Answer from the drawing. Dimensions are ordinates in mm from the lowest x, y and z of the part. A direction names the side the tool comes from. Coordinates: 2 decimals unless noted, no trailing zeros. Write each loop counter-clockwise with the first axis right and the second up, starting at its lowest first coordinate (ties: lowest second). Pieces come first, ordered by that corner, then holes. Notation, with made-up numbers: (22.5, -9.75) -> (54.5, -9.75) arc R24 cw to (54.5, 6.25) -> close; hole circle Ø4 at (55, 47). An arc over 180 degrees is marked (long way). Answer as a JSON object with one key per item and string values. Group by question number.
(1) Which of the six approach directions +Z, -Z, +X, -X, +Y, -Y give full straight-line access (tool end or side, diameter ignored) to the marked faces 1, 2 and 3?
(2) Straight lines are drawn through the part: L1, parallel to Z at x = 10, y = 19; L2, parallel to X at y = 22, z = 10; L3, parallel to Y at x = 10, z = 6. For each, find the intervals that lie inside material, in ascending order.
(3) For a pull along X with two mould halves and no side action, classify the marked faces 4, 5 and 6 as +X half, -X half, draft (parallel to the pull), parting line (faces both ways), or undercut.
(4) Find section D-D (y = 7.25). Give the vertices of the cut face in (x, z).
(5) Find section B-B (z = 5.5). Give the vertices of the cut face in (x, y), then the cut area to 3 significant figures.
(6) Find section C-C (x = 18). Give the vertices of the cut face in (y, z), then the cut area to 3 significant figures.
(7) Find section A-A (y = 21.5). Give the vertices of the cut face in (x, z) (1 decimal).
(8) Flat-ended cylindrical pins translate along their axes: P1, Ø3, axis at x = 10, y = 22, coming from the -Z side; P2, Ø2, axis at x = 11, z = 9, coming from the +Y side; P3, Ø1.2, axis at x = 10, y = 21.5, coming from the -Z side; P4, Ø6, axis at y = 22, z = 4, coming from the -X side (1 decimal). Find the tip coordinate at first contact, or state that the pin passes through.
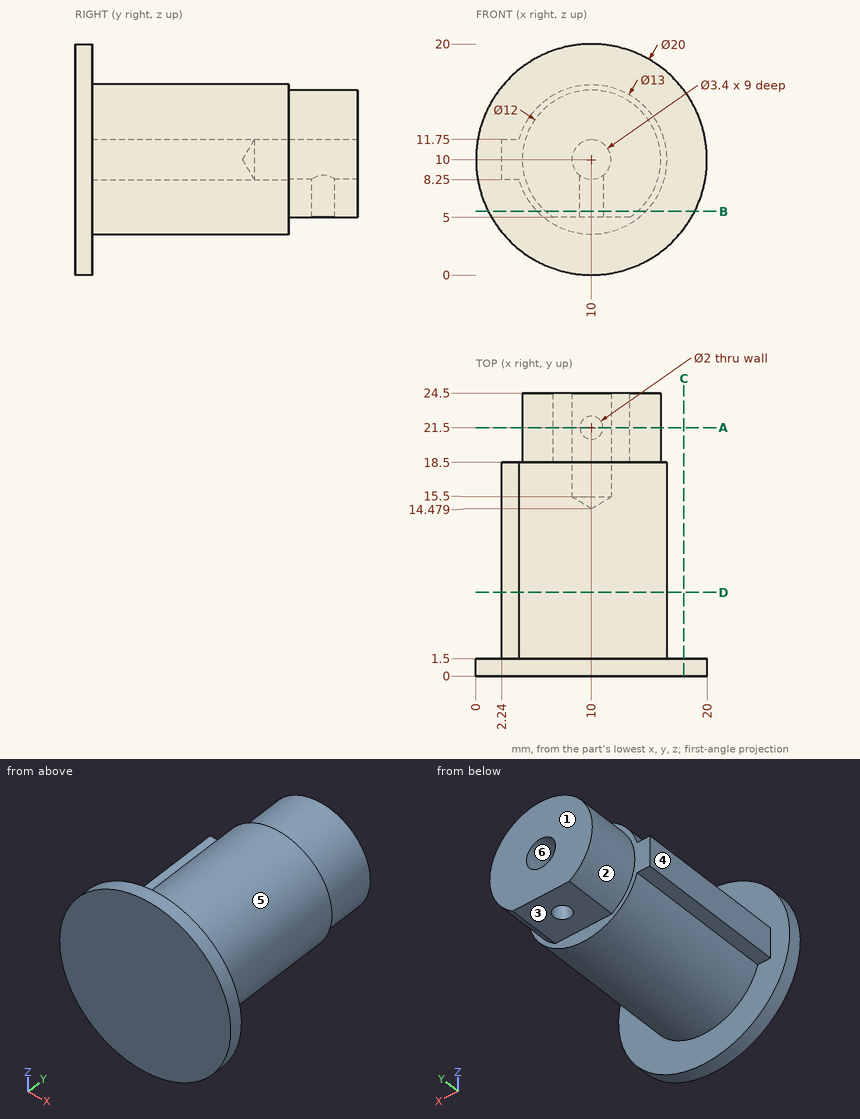
Results below:
{
 "1": {"face 1": "+Z, -Z, +X, -X, +Y", "face 2": "+Y", "face 3": "-Z, +X, -X, +Y"},
 "2": {"L1": "z = 5 to 8.3, 11.7 to 16", "L2": "x = 4 to 8.3, 11.7 to 16", "L3": "y = 0 to 20.5, 22.5 to 24.5"},
 "3": {"face 4": "-X half", "face 5": "parting line", "face 6": "undercut"},
 "4": {"outline": "(2.24, 8.25) -> (3.74, 8.25) arc R6.5 ccw (long way) to (3.74, 11.75) -> (2.24, 11.75) -> close"},
 "5": {"outline": "(1.07, 0) -> (18.93, 0) -> (18.93, 1.5) -> (14.69, 1.5) -> (14.69, 18.5) -> (13.97, 18.5) -> (13.97, 24.5) -> (6.03, 24.5) -> (6.03, 18.5) -> (5.31, 18.5) -> (5.31, 1.5) -> (1.07, 1.5) -> close; hole circle Ø2 at (10, 21.5)", "area": "231 mm2"},
 "6": {"outline": "(0, 4) -> (1.5, 4) -> (1.5, 16) -> (0, 16) -> close", "area": "18.0 mm2"},
 "7": {"outline": "(6.7, 5) -> (9, 5) -> (9, 8.6) arc R1.7 cw (long way) to (11, 8.6) -> (11, 5) -> (13.3, 5) arc R6 ccw (long way) to start"},
 "8": {"P1": "stops at z = 5", "P2": "stops at y = 24.5", "P3": "stops at z = 11.59", "P4": "stops at x = 4.8"}
}
